from build123d import *

# Parameters (mm, degrees)
ESBO_O1_W              = 22.5
ESBO_O1_H              = 12
BODY_DEPTH             = 4.7
BODY_DEPTH_BACK        = 18
TABS_DEPTH             = 2.375
TOP_GEAR_HOUSING_DEPTH = 4
ESBO_O4_R              = 2.25
SHAFT_DEPTH            = 3
ESBO_O5_R              = 0.75
SHAFT_HOLE_DEPTH       = 5
FILETE2_R              = 0.5
SKETCH1_R              = 0.5
BOSS_EXTRUDE1_DEPTH    = 10
LPATTERN2_COUNT        = 3
LPATTERN2_PITCH        = 1.001


with BuildPart() as part:
    # Esbo_o1 → Body (new body, two sides)
    with BuildSketch(Plane(origin=(0, 0, 0), x_dir=(1, 0, 0), z_dir=(0, 1, 0))) as body_sk:
        Rectangle(ESBO_O1_W, ESBO_O1_H)
    extrude(amount=BODY_DEPTH)
    extrude(body_sk.sketch, amount=-BODY_DEPTH_BACK)

    # Esbo_o2 → tabs (add)
    with BuildSketch(Plane(origin=(0, 0, 0), x_dir=(1, 0, 0), z_dir=(0, 1, 0))):
        with BuildLine():
            Line((-11.25, 6), (-16.21, 6))
            Line((-16.21, 6), (-16.21, 0.5))
            Line((-16.21, 0.5), (-14.954795897, 0.5))
            ThreePointArc((-14.954795897, 0.5), (-12.875, 0), (-14.954795897, -0.5))
            Line((-14.954795897, -0.5), (-16.21, -0.5))
            Line((-16.21, -0.5), (-16.21, -6))
            Line((-16.21, -6), (-11.25, -6))
            Line((-11.25, -6), (-11.25, 6))
        make_face()
        with BuildLine():
            Line((11.25, 6), (16.21, 6))
            Line((16.21, 6), (16.21, 0.5))
            Line((16.21, 0.5), (14.709795897, 0.5))
            ThreePointArc((14.709795897, 0.5), (12.63, 0), (14.709795897, -0.5))
            Line((14.709795897, -0.5), (16.21, -0.5))
            Line((16.21, -0.5), (16.21, -6))
            Line((16.21, -6), (11.25, -6))
            Line((11.25, -6), (11.25, 6))
        make_face()
    extrude(amount=-TABS_DEPTH)

    # Esbo_o3 → Top Gear Housing (add)
    with BuildSketch(Plane(origin=(0, 4.7, 0), x_dir=(1, 0, 0), z_dir=(0, 1, 0))):
        with BuildLine():
            Line((0.029914772, 2.85), (1.25, 2.85))
            ThreePointArc((1.25, 2.85), (4.1, 0), (1.25, -2.85))
            Line((1.25, -2.85), (0.029914772, -2.85))
            ThreePointArc((0.029914772, -2.85), (-11.25, 0), (0.029914772, 2.85))
        make_face()
    extrude(amount=TOP_GEAR_HOUSING_DEPTH)

    # Esbo_o4 → shaft (add)
    with BuildSketch(Plane(origin=(0, 8.7, 0), x_dir=(1, 0, 0), z_dir=(0, 1, 0))):
        with Locations((-5.25, 0)):
            Circle(ESBO_O4_R)
    extrude(amount=SHAFT_DEPTH)

    # Esbo_o5 → shaft hole (cut)
    with BuildSketch(Plane(origin=(0, 11.7, 0), x_dir=(1, 0, 0), z_dir=(0, 1, 0))):
        with Locations((-5.25, 0)):
            Circle(ESBO_O5_R)
    extrude(amount=-SHAFT_HOLE_DEPTH, mode=Mode.SUBTRACT)

    # Filete2
    filete2_edges = [part.edges().sort_by_distance(p)[0] for p in [
        (-11.25, 8.7, 0),
        (0.639957386, 8.7, 2.85),
        (4.1, 8.7, 0),
        (0.639957386, 8.7, -2.85),
    ]]
    fillet(filete2_edges, radius=FILETE2_R)

    # Sketch1 → Boss-Extrude1 (add)
    with BuildSketch(Plane.ZY.offset(11.25)):
        with Locations((-1, -12.875)):
            Circle(SKETCH1_R)
    boss_extrude1 = extrude(amount=BOSS_EXTRUDE1_DEPTH)

    # LPattern2: Boss-Extrude1 ×3
    with Locations(*[(0, 0, i * LPATTERN2_PITCH) for i in range(1, LPATTERN2_COUNT)]):
        add(boss_extrude1)


solid = part.part
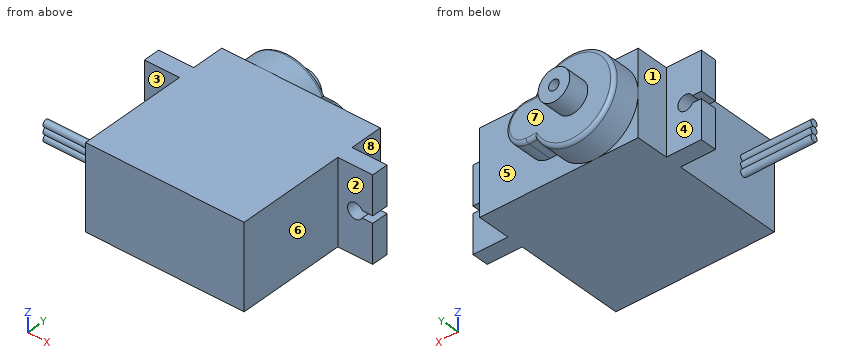
Design review of the part built by this model. Coordinates are the model's own, in mm. Face numbers are marked on the shaded views. A direction names the side the tool comes from. Coordinates: 2 decimals unless noted, no trailing zeros. Loops run counter-clockwise (first coordinate to the right, second up) from the corner with the lowest first, then second, coordinate; pieces in that order, holes last. Notation, with made-up numbers: (-20, 47) -> (37, 47) arc R38 ccw to (37, 85) -> close; hole circle Ø3 at (79, 66.25). An arc over 180 degrees is marked (long way). Use a Markdown table: item, result. Add a question column.
Item 1: Machinability: for the marked faces 5, 6, 7 and 8, which of the approach directions +Z, -Z, +X, -X, +Y, -Y give a long, thin tool a straight path to every point of the face, cutting with its end or side? Answer none if there is none.
Item 2: We need section C-C, the plane y = -0.5. Write out the cut boundary in (x, z) (3 decimals).
Item 3: We need section B-B, the plane x = 13.73. Write out the cut boundary in (y, z) (3 decimals).
Item 4: The part is to be moulded in two halves that separate along Y. For the marked faces 1, 2, 3 and 4, say which applies: +Y half, -Y half, draft (parallel to the pull), parting line (faces both ways), or undercut.
Item 5: We need section A-A, the plane x = -15.5. Write out the cut boundary in (y, z) (3 decimals), and give its area (3 significant figures).
Item 6: Wall thickness on L1, parallel to X at y = 9.8, z = 0; L2, parallel to Z at x = -5.25, y = 8.2; L3, parallel to Z at x = 13.73, y = -1.85: over which ranges is each line inside the solid? List them lowest first. Write a range as from..to.
Item 7: We need section D-D, the plane y = -6.5. Write out the cut boundary in (x, z), and give its area (3 significant figures).
Item 8: Clearance check with flat-ended pins moving along their axes: P1, Ø3.5, axis at x = -1, z = 1.5, coming from the +Y side; P2, Ø4, axis at x = 13, z = -2, coming from the +Y side; P3, Ø1, axis at x = 0.5, y = 6, coming from the -Z side; P4, Ø2, axis at x = 13.73, z = 0, coming from the -Y side. State where each tip first meets the part, or that it passes through.
Numbers:
| question | item | result |
|---|---|---|
| 1 | face 5 | +X, +Y |
| 1 | face 6 | +Z, -Z, +X, -Y |
| 1 | face 7 | +Y |
| 1 | face 8 | +Z, -Z, +X, +Y |
| 2 | outline | (-16.21, -6) -> (16.21, -6) -> (16.21, -0.5) -> (14.71, -0.5) arc R1.1 cw (long way) to (14.71, 0.5) -> (16.21, 0.5) -> (16.21, 6) -> (-16.21, 6) -> (-16.21, 0.5) -> (-14.955, 0.5) arc R1.1 cw (long way) to (-14.955, -0.5) -> (-16.21, -0.5) -> close |
| 3 | outline | (-2.375, -6) -> (0, -6) -> (0, -1.1) -> (-2.375, -1.1) -> close; (-2.375, 1.1) -> (0, 1.1) -> (0, 6) -> (-2.375, 6) -> close |
| 4 | face 1 | draft |
| 4 | face 2 | -Y half |
| 4 | face 3 | undercut |
| 4 | face 4 | +Y half |
| 5 | outline | circle Ø1 at (-12.875, -1); circle Ø1 at (-12.875, 0.001); circle Ø1 at (-12.875, 1.002); (-2.375, -6) -> (0, -6) -> (0, -0.5) -> (-2.375, -0.5) -> close; (-2.375, 0.5) -> (0, 0.5) -> (0, 6) -> (-2.375, 6) -> close |
| 5 | area | 28.5 mm^2 |
| 6 | L1 | x = -7.5..-6, -4.5..-3 |
| 6 | L2 | z = -6..-0.75, 0.75..6 |
| 6 | L3 | z = -6..-1.1, 1.1..6 |
| 7 | outline | (-11.25, -6) -> (11.25, -6) -> (11.25, 6) -> (-11.25, 6) -> close |
| 7 | area | 270 mm^2 |
| 8 | P1 | stops at y = 8.7 |
| 8 | P2 | stops at y = 4.7 |
| 8 | P3 | stops at z = -2.9 |
| 8 | P4 | passes through |
